For this review, take the finished solid that the model builds, in its own axes (mm). A direction names the side the tool comes from. Give positions to 0.01 mm unless a question says otherwise; leave off trailing zeros. Loops run counter-clockwise (first coordinate to the right, second up) from the corner with the lowest first, then second, coordinate; pieces in that order, holes last.
```python
from build123d import *

# Parameters (mm, degrees)
EXTRUDE_1_DEPTH             = 40
SKETCH_2_R                  = 7.25
CUT_EXTRUDE_1_DEPTH         = 1
CHAMFER_1_SIZE              = 0.5
SKETCH_5_R                  = 5.5
CUT_EXTRUDE_2_DEPTH         = 1
CHAMFER_2_SIZE              = 0.5
CHAMFER_2_SIZE2             = 0.288675135
SKETCH_6_R                  = 4.5
CUT_EXTRUDE_3_DEPTH         = 1
CHAMFER_3_SIZE              = 0.5
CHAMFER_3_SIZE2             = 0.866025404
SKETCH_7_R                  = 2.5
CUT_EXTRUDE_4_DEPTH         = 1
CHAMFER_4_SIZE              = 0.5
CHAMFER_4_SIZE2             = 0.866025404
CHAMFER_1_OF_MIRROR_3_SIZE  = 0.5
CHAMFER_2_OF_MIRROR_3_SIZE2 = 0.288675135
CHAMFER_2_OF_MIRROR_3_SIZE  = 0.5
CHAMFER_3_OF_MIRROR_3_SIZE2 = 0.866025404
CHAMFER_3_OF_MIRROR_3_SIZE  = 0.5
CHAMFER_4_OF_MIRROR_3_SIZE2 = 0.5
CHAMFER_4_OF_MIRROR_3_SIZE  = 0.866025404
SKETCH_9_R                  = 7.25
CUT_EXTRUDE_5_DEPTH         = 1
CHAMFER_5_SIZE              = 0.5
SKETCH_10_R                 = 5.6
CUT_EXTRUDE_6_DEPTH         = 1
CHAMFER_6_SIZE              = 0.5
CHAMFER_6_SIZE2             = 0.866025404
SKETCH_11_R                 = 4.35
CUT_EXTRUDE_7_DEPTH         = 1
CHAMFER_7_SIZE              = 0.5
CHAMFER_7_SIZE2             = 0.866025404
SKETCH_12_R                 = 3
CUT_EXTRUDE_8_DEPTH         = 1
CHAMFER_8_SIZE              = 0.5
CHAMFER_8_SIZE2             = 0.866025404
CUT_EXTRUDE_9_DEPTH         = 1.5
FILLET_1_R                  = 1
SKETCH_14_R                 = 2
CUT_EXTRUDE_10_DEPTH        = 1
FILLET_2_R                  = 0.6
SKETCH_15_R                 = 2
CUT_EXTRUDE_11_DEPTH        = 1
FILLET_3_R                  = 0.6
CUT_EXTRUDE_12_DEPTH        = 3
SKETCH_17_W                 = 26
SKETCH_17_H                 = 7
EXTRUDE_2_DEPTH             = 6.5
SKETCH_18_W                 = 6.5
SKETCH_18_H                 = 5
SKETCH_18_W_2               = 5
CUT_EXTRUDE_13_DEPTH        = 3
SKETCH_19_R                 = 1.25
CUT_EXTRUDE_14_DEPTH        = 3


with BuildPart() as part:
    # 草图1 → 凸台-拉伸1 (new body)
    with BuildSketch(Plane.XY):
        with BuildLine():
            Line((-64.7, 15), (70.15, 15))
            ThreePointArc((70.15, 15), (85.15, 0), (70.15, -15))
            Line((70.15, -15), (-64.7, -15))
            ThreePointArc((-64.7, -15), (-79.7, 0), (-64.7, 15))
        make_face()
    extrude(amount=EXTRUDE_1_DEPTH)

    # 草图2 → 切除-拉伸1 (cut)
    with BuildSketch(Plane(origin=(0, 0, 0), x_dir=(-1, 0, 0), z_dir=(0, 0, -1))):
        with Locations((-37.5, 0)):
            Circle(SKETCH_2_R)
    cut_extrude_1 = extrude(amount=-CUT_EXTRUDE_1_DEPTH, mode=Mode.SUBTRACT)

    # 倒角1
    chamfer_1_edges = [part.edges().sort_by_distance(p)[0] for p in [
        (44.75, 0, 1),
        (44.75, 0, 0),
    ]]
    chamfer(chamfer_1_edges, length=CHAMFER_1_SIZE - 0.0001)  # a hair under: the kernel refuses the full size

    # 草图5 → 切除-拉伸2 (cut)
    with BuildSketch(Plane(origin=(0, 0, 1), x_dir=(-1, 0, 0), z_dir=(0, 0, -1))):
        with Locations((-37.5, 0)):
            Circle(SKETCH_5_R)
    cut_extrude_2 = extrude(amount=-CUT_EXTRUDE_2_DEPTH, mode=Mode.SUBTRACT)

    # 倒角2
    chamfer_2_edges = [part.edges().sort_by_distance(p)[0] for p in [
        (43, 0, 1),
    ]]
    chamfer_2_side = [part.faces().sort_by_distance(p)[0] for p in [
        (43, 0, 1.5),
    ]]
    chamfer(chamfer_2_edges, length=CHAMFER_2_SIZE, length2=CHAMFER_2_SIZE2, reference=chamfer_2_side[0])

    # 草图6 → 切除-拉伸3 (cut)
    with BuildSketch(Plane(origin=(0, 0, 2), x_dir=(-1, 0, 0), z_dir=(0, 0, -1))):
        with Locations((-37.5, 0)):
            Circle(SKETCH_6_R)
    cut_extrude_3 = extrude(amount=-CUT_EXTRUDE_3_DEPTH, mode=Mode.SUBTRACT)

    # 倒角3
    chamfer_3_edges = [part.edges().sort_by_distance(p)[0] for p in [
        (42, 0, 2),
    ]]
    chamfer_3_side = [part.faces().sort_by_distance(p)[0] for p in [
        (42, 0, 2.5),
    ]]
    chamfer(chamfer_3_edges, length=CHAMFER_3_SIZE, length2=CHAMFER_3_SIZE2, reference=chamfer_3_side[0])

    # 草图7 → 切除-拉伸4 (cut)
    with BuildSketch(Plane(origin=(0, 0, 3), x_dir=(-1, 0, 0), z_dir=(0, 0, -1))):
        with Locations((-37.5, 0)):
            Circle(SKETCH_7_R)
    cut_extrude_4 = extrude(amount=-CUT_EXTRUDE_4_DEPTH, mode=Mode.SUBTRACT)

    # 倒角4
    chamfer_4_edges = [part.edges().sort_by_distance(p)[0] for p in [
        (40, 0, 3),
    ]]
    chamfer_4_side = [part.faces().sort_by_distance(p)[0] for p in [
        (41.872720779, 0, 3),
    ]]
    chamfer(chamfer_4_edges, length=CHAMFER_4_SIZE, length2=CHAMFER_4_SIZE2, reference=chamfer_4_side[0])

    # 镜向3: 切除-拉伸1, 切除-拉伸2, 切除-拉伸3, 切除-拉伸4 across plane
    add(cut_extrude_1.mirror(Plane(origin=(0, 0, 0), x_dir=(0, 0, 1), z_dir=(1, 0, 0))), mode=Mode.SUBTRACT)
    add(cut_extrude_2.mirror(Plane(origin=(0, 0, 0), x_dir=(0, 0, 1), z_dir=(1, 0, 0))), mode=Mode.SUBTRACT)
    add(cut_extrude_3.mirror(Plane(origin=(0, 0, 0), x_dir=(0, 0, 1), z_dir=(1, 0, 0))), mode=Mode.SUBTRACT)
    add(cut_extrude_4.mirror(Plane(origin=(0, 0, 0), x_dir=(0, 0, 1), z_dir=(1, 0, 0))), mode=Mode.SUBTRACT)

    # 倒角1 of 镜向3
    chamfer_1_of_mirror_3_edges = [part.edges().sort_by_distance(p)[0] for p in [
        (-44.75, 0, 1),
        (-44.75, 0, 0),
    ]]
    chamfer(chamfer_1_of_mirror_3_edges, length=CHAMFER_1_OF_MIRROR_3_SIZE - 0.0001)  # a hair under: the kernel refuses the full size

    # 倒角2 of 镜向3
    chamfer_2_of_mirror_3_edges = [part.edges().sort_by_distance(p)[0] for p in [
        (-43, 0, 1),
    ]]
    chamfer(chamfer_2_of_mirror_3_edges, length=CHAMFER_2_OF_MIRROR_3_SIZE, length2=CHAMFER_2_OF_MIRROR_3_SIZE2)

    # 倒角3 of 镜向3
    chamfer_3_of_mirror_3_edges = [part.edges().sort_by_distance(p)[0] for p in [
        (-42, 0, 2),
    ]]
    chamfer(chamfer_3_of_mirror_3_edges, length=CHAMFER_3_OF_MIRROR_3_SIZE, length2=CHAMFER_3_OF_MIRROR_3_SIZE2)

    # 倒角4 of 镜向3
    chamfer_4_of_mirror_3_edges = [part.edges().sort_by_distance(p)[0] for p in [
        (-40, 0, 3),
    ]]
    chamfer(chamfer_4_of_mirror_3_edges, length=CHAMFER_4_OF_MIRROR_3_SIZE, length2=CHAMFER_4_OF_MIRROR_3_SIZE2)

    # 草图9 → 切除-拉伸5 (cut)
    with BuildSketch(Plane(origin=(0, 0, 0), x_dir=(-1, 0, 0), z_dir=(0, 0, -1))):
        with Locations((12.5, 0)):
            Circle(SKETCH_9_R)
    extrude(amount=-CUT_EXTRUDE_5_DEPTH, mode=Mode.SUBTRACT)

    # 倒角5
    chamfer_5_edges = [part.edges().sort_by_distance(p)[0] for p in [
        (-5.25, 0, 1),
    ]]
    chamfer(chamfer_5_edges, length=CHAMFER_5_SIZE)

    # 草图10 → 切除-拉伸6 (cut)
    with BuildSketch(Plane(origin=(0, 0, 1), x_dir=(-1, 0, 0), z_dir=(0, 0, -1))):
        with Locations((12.5, 0)):
            Circle(SKETCH_10_R)
    extrude(amount=-CUT_EXTRUDE_6_DEPTH, mode=Mode.SUBTRACT)

    # 倒角6
    chamfer_6_edges = [part.edges().sort_by_distance(p)[0] for p in [
        (-6.9, 0, 1),
    ]]
    chamfer_6_side = [part.faces().sort_by_distance(p)[0] for p in [
        (-6.9, 0, 1.5),
    ]]
    chamfer(chamfer_6_edges, length=CHAMFER_6_SIZE, length2=CHAMFER_6_SIZE2, reference=chamfer_6_side[0])

    # 草图11 → 切除-拉伸7 (cut)
    with BuildSketch(Plane(origin=(0, 0, 2), x_dir=(-1, 0, 0), z_dir=(0, 0, -1))):
        with Locations((12.5, 0)):
            Circle(SKETCH_11_R)
    extrude(amount=-CUT_EXTRUDE_7_DEPTH, mode=Mode.SUBTRACT)

    # 倒角7
    chamfer_7_edges = [part.edges().sort_by_distance(p)[0] for p in [
        (-8.15, 0, 2),
    ]]
    chamfer_7_side = [part.faces().sort_by_distance(p)[0] for p in [
        (-8.15, 0, 2.5),
    ]]
    chamfer(chamfer_7_edges, length=CHAMFER_7_SIZE, length2=CHAMFER_7_SIZE2, reference=chamfer_7_side[0])

    # 草图12 → 切除-拉伸8 (cut)
    with BuildSketch(Plane(origin=(0, 0, 3), x_dir=(-1, 0, 0), z_dir=(0, 0, -1))):
        with Locations((12.5, 0)):
            Circle(SKETCH_12_R)
    extrude(amount=-CUT_EXTRUDE_8_DEPTH, mode=Mode.SUBTRACT)

    # 倒角8
    chamfer_8_edges = [part.edges().sort_by_distance(p)[0] for p in [
        (-9.5, 0, 4),
    ]]
    chamfer_8_side = [part.faces().sort_by_distance(p)[0] for p in [
        (-9.5, 0, 3.5),
    ]]
    chamfer(chamfer_8_edges, length=CHAMFER_8_SIZE, length2=CHAMFER_8_SIZE2, reference=chamfer_8_side[0])

    # 草图13 → 切除-拉伸9 (cut)
    with BuildSketch(Plane(origin=(0, 0, 0), x_dir=(-1, 0, 0), z_dir=(0, 0, -1))):
        with BuildLine():
            Line((-70.249806967, 12.989941679), (64.685358142, 12.989941679))
            ThreePointArc((64.685358142, 12.989941679), (77.675299821, 0), (64.685358142, -12.989941679))
            Line((64.685358142, -12.989941679), (-70.249806967, -12.989941679))
            ThreePointArc((-70.249806967, -12.989941679), (-83.239748646, 0), (-70.249806967, 12.989941679))
        make_face()
    extrude(amount=-CUT_EXTRUDE_9_DEPTH, mode=Mode.SUBTRACT)

    # 圆角1
    fillet_1_edges = [part.edges().sort_by_distance(p)[0] for p in [
        (83.239748646, 0, 1.5),
        (2.782224413, 12.989941679, 1.5),
        (-77.675299821, 0, 1.5),
        (2.782224413, -12.989941679, 1.5),
    ]]
    fillet(fillet_1_edges, radius=FILLET_1_R)

    # 草图14 → 切除-拉伸10 (cut)
    with BuildSketch(Plane(origin=(0, 0, 1.5), x_dir=(-1, 0, 0), z_dir=(0, 0, -1))):
        with Locations((-24.5, 4.5)):
            Circle(SKETCH_14_R)
    extrude(amount=-CUT_EXTRUDE_10_DEPTH, mode=Mode.SUBTRACT)

    # 圆角2
    fillet_2_edges = [part.edges().sort_by_distance(p)[0] for p in [
        (26.5, 4.5, 2.5),
    ]]
    fillet(fillet_2_edges, radius=FILLET_2_R)

    # 草图15 → 切除-拉伸11 (cut)
    with BuildSketch(Plane(origin=(0, 0, 1.5), x_dir=(-1, 0, 0), z_dir=(0, 0, -1))):
        with Locations((-24.5, -4.5)):
            Circle(SKETCH_15_R)
    extrude(amount=-CUT_EXTRUDE_11_DEPTH, mode=Mode.SUBTRACT)

    # 圆角3
    fillet_3_edges = [part.edges().sort_by_distance(p)[0] for p in [
        (26.5, -4.5, 2.5),
    ]]
    fillet(fillet_3_edges, radius=FILLET_3_R)

    # 草图16 → 切除-拉伸12 (cut)
    with BuildSketch(Plane(origin=(0, 0, 1.5), x_dir=(-1, 0, 0), z_dir=(0, 0, -1))):
        with BuildLine():
            ThreePointArc((-59.831299631, 1.114743341), (-60.893840639, -0.011454355), (-59.767642942, -1.073995363))
            ThreePointArc((-59.767642942, -1.073995363), (-59.385256659, -0.668700369), (-59.790551653, -0.286314086))
            ThreePointArc((-59.790551653, -0.286314086), (-60.106159361, 0.011454355), (-59.80839092, 0.327062064))
            ThreePointArc((-59.80839092, 0.327062064), (-59.426004637, 0.732357058), (-59.831299631, 1.114743341))
        make_face()
    cut_extrude_12 = extrude(amount=-CUT_EXTRUDE_12_DEPTH, mode=Mode.SUBTRACT)

    # 镜向6: 切除-拉伸12 across plane
    add(cut_extrude_12.mirror(Plane(origin=(0, 0, 0), x_dir=(0, 0, 1), z_dir=(1, 0, 0))), mode=Mode.SUBTRACT)

    # 草图17 → 凸台-拉伸2 (add)
    with BuildSketch(Plane.XZ.offset(15)):
        with Locations((0, 10.5)):
            Rectangle(SKETCH_17_W, SKETCH_17_H)
    extrude(amount=EXTRUDE_2_DEPTH)

    # 草图18 → 切除-拉伸13 (cut)
    with BuildSketch(Plane.XZ.offset(21.5)):
        with Locations((-9.75, 10.5)):
            Rectangle(SKETCH_18_W, SKETCH_18_H)
        with Locations((9.75, 10.5)):
            Rectangle(SKETCH_18_W, SKETCH_18_H)
        with Locations((-3, 10.5)):
            Rectangle(SKETCH_18_W_2, SKETCH_18_H)
        with Locations((3, 10.5)):
            Rectangle(SKETCH_18_W_2, SKETCH_18_H)
    extrude(amount=-CUT_EXTRUDE_13_DEPTH, mode=Mode.SUBTRACT)

    # 草图19 → 切除-拉伸14 (cut)
    with BuildSketch(Plane.XZ.offset(18.5)):
        with Locations(Location((9, 11, 0), (0, 0, 270))):
            Circle(SKETCH_19_R)
        with Locations(Location((-9.7, 11, 0), (0, 0, 270))):
            Circle(SKETCH_19_R)
    extrude(amount=-CUT_EXTRUDE_14_DEPTH, mode=Mode.SUBTRACT)


solid = part.part
```
Q1. Consider section C-C on x = 24.5. Give the boundary of the cut face in (y, z).
Answers:
outline: (-15, 0) - (-12.99, 0) - (-12.99, 0.5) arc R1 cw to (-11.99, 1.5) - (-6.5, 1.5) - (-6.5, 1.9) arc R0.6 cw to (-5.9, 2.5) - (-3.1, 2.5) arc R0.6 cw to (-2.5, 1.9) - (-2.5, 1.5) - (2.5, 1.5) - (2.5, 1.9) arc R0.6 cw to (3.1, 2.5) - (5.9, 2.5) arc R0.6 cw to (6.5, 1.9) - (6.5, 1.5) - (11.99, 1.5) arc R1 cw to (12.99, 0.5) - (12.99, 0) - (15, 0) - (15, 40) - (-15, 40) - close
Q2. For pin 1 Ø5.5 at (x, y) = (37.5, 0) entering from -Z; pin 2 Ø4.5 at (x, y) = (-13.5, 0) entering from -Z; pin 3 Ø1.5 at (x, y) = (-10, -20.5) entering from +Z, all flat-tipped, find the tip position at first contact; note any pin that passes through.
Answers:
pin 1: stops at z = 3.43
pin 2: stops at z = 3
pin 3: stops at z = 14
Q3. Mouldability with a two-part tool opening along Y and no side actions: class faces 1 (the flat face through (10, -20, 13)), 2 (the cylindrical face through (85.146, 0.33, 19.72)), 3 (the cylindrical face through (-35.19, -0.96, 3.75)), 4 (the flat face through (10.4, -18.5, 10.5)) as +Y half, -Y half, draft (parallel to the pull), parting line (faces both ways), or undercut.
Answers:
face 1: draft
face 2: parting line
face 3: undercut
face 4: -Y half
Q4. Consider section A-A on x = 3.5. Give the boundary of the cut face in (y, z).
Answers:
outline: (-21.5, 7) - (-15, 7) - (-15, 0) - (-12.99, 0) - (-12.99, 0.5) arc R1 cw to (-11.99, 1.5) - (11.99, 1.5) arc R1 cw to (12.99, 0.5) - (12.99, 0) - (15, 0) - (15, 40) - (-15, 40) - (-15, 14) - (-21.5, 14) - (-21.5, 13) - (-18.5, 13) - (-18.5, 8) - (-21.5, 8) - close
Q5. Consider section B-B on y = -17. Give the boundary of the cut face in (x, z), plus the area to 3 significant figures.
Answers:
outline: (-13, 7) - (13, 7) - (13, 14) - (-13, 14) - close; hole circle Ø2.5 at (-9.7, 11); hole circle Ø2.5 at (9, 11)
area: 172 mm2
Q6. For probe 1 along Y at (x, z) = (24.5, 1.75); probe 2 along Z at (x, y) = (12, 4); probe 3 along Y at (x, z) = (43, 23), list the stretches that pass through material, from the lowest coordinate up.
Answers:
probe 1: y = -15 to -6.5, -2.5 to 2.5, 6.5 to 15
probe 2: z = 1.5 to 40
probe 3: y = -15 to 15
Q7. Consider section D-D on z = 23. Give the boundary of the cut face in (x, y), plus the area to 3 significant figures.
Answers:
outline: (-64.7, -15) - (70.15, -15) arc R15 ccw to (70.15, 15) - (-64.7, 15) arc R15 ccw to start
area: 4,750 mm2
Q8. Machinability: for faces 5 (the flat face through (0, -18, 14)), 6 (the flat face through (-11, -3, 3)), 7 (the flat face through (-6.5, -20, 10)), which of the approach directions +Z, -Z, +X, -X, +Y, -Y give a long, thin tool a straight path to every point of the face, cutting with its end or side? Answer none if there is none.
Answers:
face 5: +Z, +X, -X, -Y
face 6: -Z
face 7: -X, -Y
